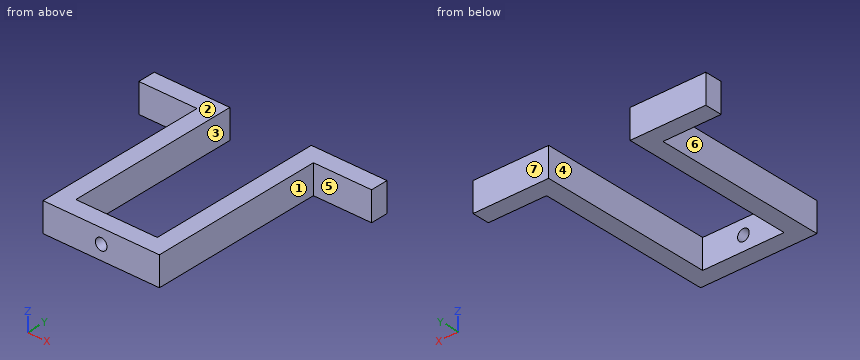
```python
from build123d import *

# Parameters (mm, degrees)
PAD_DEPTH         = 5
SKETCH001_R       = 1
POCKET_DEPTH      = 30.001
POCKET_DEPTH_BACK = -3.001


with BuildPart() as part:
    # Sketch → Pad (new body)
    with BuildSketch(Plane.XY):
        Polygon((7, 0), (-7, 0), (-7, 30), (-20, 30), (-20, 27), (-10, 27), (-10, -3), (10, -3), (10, 27), (20, 27), (20, 30), (7, 30), align=None)
    extrude(amount=PAD_DEPTH)

    # Sketch001 → Pocket (cut, two sides)
    with BuildSketch(Plane.XZ) as pocket_sk:
        with Locations((0, 2.5)):
            Circle(SKETCH001_R)
    extrude(amount=-POCKET_DEPTH, mode=Mode.SUBTRACT)
    extrude(pocket_sk.sketch, amount=-POCKET_DEPTH_BACK, mode=Mode.SUBTRACT)


solid = part.part
```
Work out the finished part from the listing and answer in its coordinate system (mm). Face numbers are marked on the shaded views. A direction names the side the tool comes from. Give positions to 0.01 mm unless a question says otherwise; leave off trailing zeros. Loops run counter-clockwise (first coordinate to the right, second up) from the corner with the lowest first, then second, coordinate; pieces in that order, holes last. Notation, with made-up numbers: (66, 55.25) -> (109, 55.25) arc R26 cw to (109, 77.25) -> close; hole circle Ø11 at (55, -38). An arc over 180 degrees is marked (long way). Put each result on its own line as item: value. Start each with the question number.
Item 1: Find the intervals of material crossed by L1, parallel to X at y = -2.15, z = 2.5; L2, parallel to Z at x = 0, y = -1; L3, parallel to X at y = 16, z = 2.05, in increasing order. Write a range as [from, to].
Item 2: The mould has two halves that part along X. Classify the marked faces 1, 2 and 3: released by +X, released by -X, zero draft, split by the parting line, or undercut.
Item 3: The part is cut by section A-A (x = 0). Give the vertices of the cut face in (y, z).
Item 4: The part is cut by section D-D (x = -13). Give the vertices of the cut face in (y, z), then the cut area to 3 significant figures.
Item 5: The part is cut by section C-C (y = 12). Give the vertices of the cut face in (x, z), then the cut area to 3 significant figures.
Item 6: Which of the six approach directions +Z, -Z, +X, -X, +Y, -Y give full straight-line access (tool end or side, diameter ignored) to the marked faces 4, 5, 6 and 7?
Item 7: Each of these flat-tipped pins is pushed along its axis until it touches: P1, Ø1.8, axis at x = 0, z = 2.5, coming from the +Y side; P2, Ø1.5, axis at x = -2, z = 3, coming from the +Y side; P3, Ø2.5, axis at y = 7.5, z = 3.5, coming from the +X side; P4, Ø1.5, axis at y = 14.5, z = 1.5, coming from the -X side. Where does it stop, or does it pass through?
Item 8: The part is cut by section B-B (z = 2.5). Give the vertices of the cut face in (x, y), then the cut area to 3 significant figures.
Answers below:
1. L1: [-10, -1], [1, 10]
1. L2: [0, 1.5], [3.5, 5]
1. L3: [-10, -7], [7, 10]
2. face 1: released by +X
2. face 2: zero draft
2. face 3: undercut
3. outline: (-3, 0) -> (0, 0) -> (0, 1.5) -> (-3, 1.5) -> close; (-3, 3.5) -> (0, 3.5) -> (0, 5) -> (-3, 5) -> close
4. outline: (27, 0) -> (30, 0) -> (30, 5) -> (27, 5) -> close
4. area: 15.0 mm2
5. outline: (-10, 0) -> (-7, 0) -> (-7, 5) -> (-10, 5) -> close; (7, 0) -> (10, 0) -> (10, 5) -> (7, 5) -> close
5. area: 30.0 mm2
6. face 4: +Z, -Z, +Y
6. face 5: +Z, -Z, +X, -Y
6. face 6: +Z, -Z, -X, -Y
6. face 7: +Z, -Z, +X, -X, +Y
7. P1: through
7. P2: y = 0
7. P3: x = 10
7. P4: x = -10
8. outline: (-20, 27) -> (-10, 27) -> (-10, -3) -> (-1, -3) -> (-1, 0) -> (-7, 0) -> (-7, 30) -> (-20, 30) -> close; (1, -3) -> (10, -3) -> (10, 27) -> (20, 27) -> (20, 30) -> (7, 30) -> (7, 0) -> (1, 0) -> close
8. area: 294 mm2
